Autodesk Inventor part; units mm, degrees
ref_plane "YZ Plane" through (0, 0, 0) normal (1, 0, 0) x (0, 1, 0)
ref_plane "XZ Plane" through (0, 0, 0) normal (0, 1, 0) x (-1, 0, 0)
ref_plane "XY Plane" through (0, 0, 0) normal (0, 0, 1) x (1, 0, 0)
sketch "Sketch1" plane through (0, 0, 0) normal (0, 0, 1) x (1, 0, 0)
  arc A0 (13, 0) -> (-13, 0) centre (0, 0) ccw
  circle A1 centre (0, 0) radius 4
  line L0 (0, 13) -> (0, -20) construction
  line L1 (-13, 0) -> (-13, -20)
  line L2 (-13, -20) -> (13, -20)
  line L3 (13, -20) -> (13, 0)
  circle A2 centre (8.5, 0) radius 1.6
  circle A3 centre (-8.5, 0) radius 1.6
  line L4 (-13, -18.5) -> (13, -18.5)
  dimension "d1" = 13
  dimension "d2" = 33
  dimension "d3" = 3.2
  dimension "d4" = 8.5
  dimension "d5" = 8
  dimension "d6" = 1.5
extrude "Extrusion1" add sketch "Sketch1" along normal blind 1.5 contours L3 L4 L1 A0
extrude "Extrusion2" add sketch "Sketch1" along normal blind 32.5 contours L3 L2 L1 L4
fillet "Fillet1" radius 1.5 3 edges at (-13, -19.25, 32.5) (13, -19.25, 32.5) (0, -20, 0)
sketch "Sketch2" plane through (-13, -20, 1.5) normal (0, -1, 0) x (1, 0, 0)
  line L0 (26, 0) -> (0, 0)
  line L1 (0, 0) -> (0, 29.5)
  line L2 (24.5, 31) -> (1.5, 31)
  line L3 (13, 31) -> (13, 0) construction
  circle A0 centre (13, 16) radius 5
  circle A1 centre (21, 23) radius 2
  line L4 (21, 23) -> (21, 9) construction
  circle A2 centre (21, 9) radius 2
  circle A3 centre (5, 23) radius 2
  circle A4 centre (5, 9) radius 2
  line L5 (26, 0) -> (26, 29.5)
  point P0 (13, -1.5)
  dimension "d20" = 10
  dimension "d21" = 15
  dimension "d22" = 4
  dimension "d23" = 8
  dimension "d24" = 14
  dimension "d25" = 4
  dimension "d26" = 7
  dimension "d27" = 8
  dimension "d28" = 5
extrude "Extrusion3" cut sketch "Sketch2" against normal through all
properties part number "WH-Bracket-JGA25A"
The listing builds one solid part. Answer for the finished solid, in the listing's coordinates (mm). A direction names the side the tool comes from. Give positions to 0.01 mm unless a question says otherwise; leave off trailing zeros. Order: outer loops, then holes, each group sorted by start corner. A loop starts at its lowest first (then second) coordinate and runs counter-clockwise, first axis right, second up. Notation, with made-up numbers: (44, 31.5) -> (51, 31.5) arc R14 ccw to (51, 35.5) -> close; hole circle Ø8 at (5.5, 7.25). An arc over 180 degrees is marked (long way). Answer as a JSON object with one key per item and string values. Group by question number.
Item 1: The part is cut by section D-D on x = -8.5. Write down the section's boundary in (y, z), and give its area (3 significant figures).
Item 2: Flat-ended cylindrical pins translate along their axes: pin 1 (4 mm diameter, centred on x = -6.5, z = 10, fed in from +Y); pin 2 (4 mm diameter, centred on x = -8.5, y = 0, fed in from +Z). Find the tip coordinate at first contact, or state that the pin passes through.
Item 3: The part is cut by section A-A on z = 20.5. Write down the section's boundary in (x, y), and give its area (3 significant figures).
Item 4: The part is cut by section C-C on z = 24.5. Write down the section's boundary in (x, y), and give its area (3 significant figures).
Item 5: A tool of negligible diameter and unlimited length cuts with its end or side. For faces 1 (the flat face through (-3, -18.5, 13)), 2 (the flat face through (0, -19, 32.5)), from which of +Z, -Z, +X, -X, +Y, -Y can it reach the whole face along a straight path? Write none if from no direction.
Item 6: Consider L1, parallel to Z at x = -8, y = -19.55; L2, parallel to Z at x = -8, y = -19.15; L3, parallel to X at y = -19, z = 24. Determine where each line is inside the solid, lowest interval first. Write a range as from..to.
Item 7: The part is cut by section B-B on x = 0. Write down the section's boundary in (y, z), and give its area (3 significant figures).
Item 8: Determine the mould class of faces 3 (the flat face through (0, -6, 1.5)), 4 (the cylindrical face through (-12.55, -19.26, 32.07)), 5 (the cylindrical face through (6.9, -0.07, 0.74)) for opening direction X: pulls with the +X half, pulls with the -X half, needs draft (parallel to the pull), parting line crosses it, or undercut.
Result set:
{
 "1": {"outline": "(-20, 1.5) arc R1.5 ccw to (-18.5, 0) -> (-1.6, 0) -> (-1.6, 1.5) -> (-18.5, 1.5) -> (-18.5, 8.56) -> (-20, 8.56) -> close; (-20, 12.44) -> (-18.5, 12.44) -> (-18.5, 22.56) -> (-20, 22.56) -> close; (-20, 26.44) -> (-18.5, 26.44) -> (-18.5, 32.5) -> (-20, 32.5) -> close; (1.6, 0) -> (9.84, 0) -> (9.84, 1.5) -> (1.6, 1.5) -> close", "area": "74.4 mm²"},
 "2": {"pin 1": "y = -18.5", "pin 2": "z = 1.5"},
 "3": {"outline": "(-13, -20) -> (-4, -20) -> (-4, -18.5) -> (-13, -18.5) -> close; (4, -20) -> (13, -20) -> (13, -18.5) -> (4, -18.5) -> close", "area": "27.0 mm²"},
 "4": {"outline": "(-13, -20) -> (-10, -20) -> (-10, -18.5) -> (-13, -18.5) -> close; (-6, -20) -> (6, -20) -> (6, -18.5) -> (-6, -18.5) -> close; (10, -20) -> (13, -20) -> (13, -18.5) -> (10, -18.5) -> close", "area": "27.0 mm²"},
 "5": {"face 1": "+Z, +X, -X, +Y", "face 2": "+Z, +X, -X, +Y, -Y"},
 "6": {"L1": "0.43..8.5, 12.5..22.5, 26.5..32.5", "L2": "0.15..8.5, 12.5..22.5, 26.5..32.5", "L3": "-13..-9.94, -6.06..6.06, 9.94..13"},
 "7": {"outline": "(-20, 1.5) arc R1.5 ccw to (-18.5, 0) -> (-4, 0) -> (-4, 1.5) -> (-18.5, 1.5) -> (-18.5, 12.5) -> (-20, 12.5) -> close; (-20, 22.5) -> (-18.5, 22.5) -> (-18.5, 32.5) -> (-20, 32.5) -> close; (4, 0) -> (13, 0) -> (13, 1.5) -> (4, 1.5) -> close", "area": "68.5 mm²"},
 "8": {"face 3": "needs draft", "face 4": "pulls with the -X half", "face 5": "undercut"}
}
